Source: CAD feature listing. Evaluate the final solid. Frame: model axes, mm. Face numbers are marked on the shaded views. A direction names the side the tool comes from. Coordinates: 2 decimals unless noted, no trailing zeros. Order: outer loops, then holes, each group sorted by start corner. A loop starts at its lowest first (then second) coordinate and runs counter-clockwise, first axis right, second up. Notation, with made-up numbers: (34, 37.5) -> (92, 37.5) arc R16 ccw to (92, 63.5) -> close; hole circle Ø11 at (88.25, 0.25). An arc over 180 degrees is marked (long way). Write item = value, one per line. Start each with the question number.
Item 1: Section query C-C (x = -1.5). Output: boundary loops of the cut face in (y, z).
Item 2: Set-up query: the marked faces 1, 2 and 3. Return all of +Z, -Z, +X, -X, +Y, -Y with unobstructed straight access to the full face (end or side cutting, diameter ignored); none if empty.
Item 3: Section query D-D (y = 12). Output: boundary loops of the cut face in (x, z), then the cut area to 3 significant figures.
Item 4: Section query A-A (y = 1). Output: boundary loops of the cut face in (x, z), then the cut area to 3 significant figures.
Item 5: Mould query, pull axis X, two halves, no side actions, for the marked faces 4, 5 and 6. Classes: released by +X, released by -X, zero draft, split by the parting line, or undercut.
Item 6: Contact query for flat-ended pins moving along their axis: pin 1 (4 mm diameter, centred on y = 11.5, z = 8, fed in from +X); pin 2 (6 mm diameter, centred on y = -15.5, z = 3.5, fed in from +X); pin 3 (7 mm diameter, centred on y = 11.5, z = 5.5, fed in from -X); pin 4 (12 mm diameter, centred on x = 15.5, y = 7, fed in from -Z). Output: stop coordinate, or through.
Item 7: Ray query, line 1 along X through (y, z) = (11, 6.5); line 2 along X through (y, z) = (-15, 9.25); line 3 along Z through (x, y) = (-10, 11). Return the intervals inside material, ascending. Write a range as [from, to].
Item 8: Section query B-B (z = 5). Output: boundary loops of the cut face in (x, y).
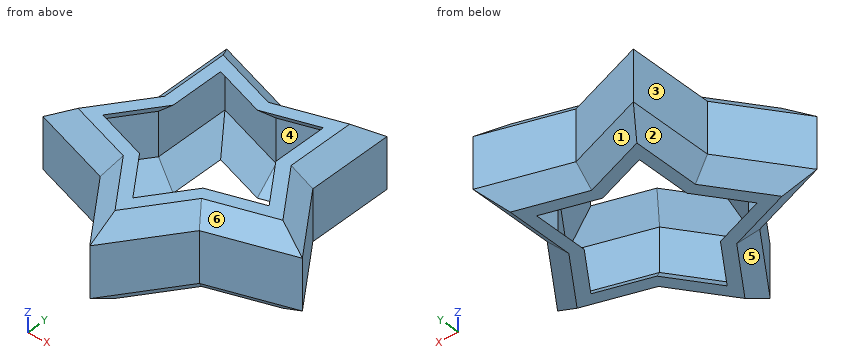
```python
from build123d import *

# Parameters (mm, degrees)
F1_DEPTH = 12.7
F2_SIZE  = 2.54
F3_T     = -1.27


with BuildPart() as f1:
    # F0 (on Top) → F1 (new body)
    with BuildSketch(Plane.XY):
        Polygon((-7.4648727041, -10.2745158286), (0, -20.5490316571), (7.4648727041, -10.2745158286), (19.5432904611, -6.35), (12.0784177569, 3.9245158286), (12.0784177569, 16.6245158286), (0, 12.7), (-12.0784177569, 16.6245158286), (-12.0784177569, 3.9245158286), (-19.5432904611, -6.35), align=None)
    extrude(amount=F1_DEPTH)

    # F2
    f2_edges = [f1.edges().sort_by_distance(p)[0] for p in [
        (-3.732436, -15.411774, 12.7),
        (3.732436, -15.411774, 12.7),
        (13.504082, -8.312258, 12.7),
        (15.810854, -1.212742, 12.7),
        (12.078418, 10.274516, 12.7),
        (6.039209, 14.662258, 12.7),
        (-6.039209, 14.662258, 12.7),
        (-12.078418, 10.274516, 12.7),
        (-15.810854, -1.212742, 12.7),
        (-13.504082, -8.312258, 12.7),
        (-13.504082, -8.312258, 0),
        (-3.732436, -15.411774, 0),
        (3.732436, -15.411774, 0),
        (13.504082, -8.312258, 0),
        (15.810854, -1.212742, 0),
        (12.078418, 10.274516, 0),
        (6.039209, 14.662258, 0),
        (-6.039209, 14.662258, 0),
        (-12.078418, 10.274516, 0),
        (-15.810854, -1.212742, 0),
    ]]
    chamfer(f2_edges, length=F2_SIZE)

    # F3
    f3_openings = [f1.faces().sort_by_distance(p)[0] for p in [
        (0, 0, 0),
        (0, 0, 12.7),
    ]]
    offset(amount=F3_T, openings=f3_openings, kind=Kind.INTERSECTION)


solid = f1.part
```
Computed:
q1.outline = (-18.48, 2.54) -> (-14.16, 0) -> (-11.11, 0) -> (-16.32, 3.07) -> (-16.32, 9.63) -> (-11.11, 12.7) -> (-14.16, 12.7) -> (-18.48, 10.16) -> close; (8.63, 0) -> (10.52, 0) -> (13.19, 2.54) -> (13.19, 10.16) -> (10.52, 12.7) -> (8.63, 12.7) -> (11.85, 9.63) -> (11.85, 3.07) -> close
q2.face_1 = -Z, +Y
q2.face_2 = -Z, -X, +Y
q2.face_3 = +Z, -Z, -X, +Y
q3.outline = (-12.08, 2.54) -> (-9.54, 0) -> (-6.07, 0) -> (0, 1.87) -> (6.07, 0) -> (9.54, 0) -> (12.08, 2.54) -> (12.08, 10.16) -> (9.54, 12.7) -> (6.07, 12.7) -> (0, 10.83) -> (-6.07, 12.7) -> (-9.54, 12.7) -> (-12.08, 10.16) -> close; hole (-10.81, 3.07) -> (-8.72, 0.98) -> (-1.96, 3.07) -> (-1.96, 9.63) -> (-8.72, 11.72) -> (-10.81, 9.63) -> close; hole (1.96, 3.07) -> (8.72, 0.98) -> (10.81, 3.07) -> (10.81, 9.63) -> (8.72, 11.72) -> (1.96, 9.63) -> close
q3.area = 118 mm^2
q4.outline = (-14.2, 2.54) -> (-11.06, 0) -> (-8.84, 0) -> (-12.63, 3.07) -> (-12.63, 9.63) -> (-8.84, 12.7) -> (-11.06, 12.7) -> (-14.2, 10.16) -> close; (8.84, 0) -> (11.06, 0) -> (14.2, 2.54) -> (14.2, 10.16) -> (11.06, 12.7) -> (8.84, 12.7) -> (12.63, 9.63) -> (12.63, 3.07) -> close
q4.area = 47.2 mm^2
q5.face_4 = undercut
q5.face_5 = released by -X
q5.face_6 = released by +X
q6.pin_1 = 12.08
q6.pin_2 = 5.85
q6.pin_3 = -12.08
q6.pin_4 = 0
q7.line_1 = [-12.08, -10.81], [10.81, 12.08]
q7.line_2 = [-4.03, -2.46], [2.46, 4.03]
q7.line_3 = [0.46, 2.26], [10.44, 12.24]
q8.outline = (-19.54, -6.35) -> (-7.46, -10.27) -> (0, -20.55) -> (7.46, -10.27) -> (19.54, -6.35) -> (12.08, 3.92) -> (12.08, 16.62) -> (0, 12.7) -> (-12.08, 16.62) -> (-12.08, 3.92) -> close; hole (-17.49, -5.68) -> (-6.68, -9.19) -> (0, -18.39) -> (6.68, -9.19) -> (17.49, -5.68) -> (10.81, 3.51) -> (10.81, 14.88) -> (0, 11.36) -> (-10.81, 14.88) -> (-10.81, 3.51) -> close
